```python
from build123d import *

# Parameters (mm, degrees)
SKETCH1_R            = 8.6
BOSS_EXTRUDE11_DEPTH = 5
SKETCH20_R           = 8.6
BOSS_EXTRUDE12_DEPTH = 5
SKETCH21_R           = 8.55
BOSS_EXTRUDE13_DEPTH = 1
SKETCH22_R           = 8.55
BOSS_EXTRUDE14_DEPTH = 7.5
SKETCH24_R           = 2.15
CUT_EXTRUDE8_DEPTH   = 7
BOSS_EXTRUDE15_START = 11.25
SKETCH30_R           = 8.55
BOSS_EXTRUDE15_DEPTH = 11.25
SKETCH31_R           = 1.6
CUT_EXTRUDE12_DEPTH  = 29.75
SKETCH32_R           = 1.5
CUT_EXTRUDE13_DEPTH  = 22.75
CIRPATTERN7_COUNT    = 2
CIRPATTERN8_COUNT    = 2
SKETCH33_R           = 2.1
CUT_EXTRUDE14_DEPTH  = 5.8
CUT_EXTRUDE15_DEPTH  = 3


with BuildPart() as part:
    # Sketch1 → Boss-Extrude11 (new body)
    with BuildSketch(Plane(origin=(0, 0, 0), x_dir=(1, 0, 0), z_dir=(0, 1, 0))):
        with Locations(Location((0, 0, 0), (0, 0, 270))):
            Circle(SKETCH1_R)
    extrude(amount=BOSS_EXTRUDE11_DEPTH)

    # Sketch20 → Boss-Extrude12 (add)
    with BuildSketch(Plane(origin=(0, 5, 0), x_dir=(1, 0, 0), z_dir=(0, 1, 0))):
        with Locations(Location((1, 0, 0), (0, 0, 93.333029494))):
            Circle(SKETCH20_R)
    extrude(amount=BOSS_EXTRUDE12_DEPTH)

    # Sketch21 → Boss-Extrude13 (add)
    with BuildSketch(Plane(origin=(0, 10, 0), x_dir=(1, 0, 0), z_dir=(0, 1, 0))):
        with Locations(Location((0.5, 0, 0), (0, 0, 94.074449123))):
            Circle(SKETCH21_R)
    extrude(amount=BOSS_EXTRUDE13_DEPTH)

    # Sketch22 → Boss-Extrude14 (add)
    with BuildSketch(Plane(origin=(0, 11, 0), x_dir=(1, 0, 0), z_dir=(0, 1, 0))):
        with Locations(Location((0.5, 0, 0), (0, 0, 94.074449123))):
            Circle(SKETCH22_R)
    extrude(amount=BOSS_EXTRUDE14_DEPTH)

    # Sketch24 → Cut-Extrude8 (cut)
    with BuildSketch(Plane(origin=(0, 18.5, 0), x_dir=(1, 0, 0), z_dir=(0, 1, 0))):
        with Locations(Location((0.7, 5, 0), (0, 0, 270))):
            Circle(SKETCH24_R)
    cut_extrude8 = extrude(amount=-CUT_EXTRUDE8_DEPTH, mode=Mode.SUBTRACT)

    # Sketch30 → Boss-Extrude15 (add)
    with BuildSketch(Plane.XZ.offset(BOSS_EXTRUDE15_START)):
        with Locations(Location((0.5, 0, 0), (0, 0, 265.925550877))):
            Circle(SKETCH30_R)
    extrude(amount=-BOSS_EXTRUDE15_DEPTH)

    # Sketch31 → Cut-Extrude12 (cut)
    with BuildSketch(Plane(origin=(0, 18.5, 0), x_dir=(1, 0, 0), z_dir=(0, 1, 0))):
        with Locations(Location((6.7, 0, 0), (0, 0, 270))):
            Circle(SKETCH31_R)
    cut_extrude12 = extrude(amount=-CUT_EXTRUDE12_DEPTH, mode=Mode.SUBTRACT)

    # Sketch32 → Cut-Extrude13 (cut)
    with BuildSketch(Plane(origin=(0, 11.5, 0), x_dir=(1, 0, 0), z_dir=(0, 1, 0))):
        with Locations(Location((0.7, 5, 0), (0, 0, 270))):
            Circle(SKETCH32_R)
    cut_extrude13 = extrude(amount=-CUT_EXTRUDE13_DEPTH, mode=Mode.SUBTRACT)

    # CirPattern7: Cut-Extrude12 ×2 about axis
    cirpattern7_axis = Axis((0.5, 0, 0), (0, 1, 0))
    for i in range(1, CIRPATTERN7_COUNT):
        add(cut_extrude12.rotate(cirpattern7_axis, i * 360 / CIRPATTERN7_COUNT), mode=Mode.SUBTRACT)

    # CirPattern8: Cut-Extrude8, Cut-Extrude13 ×2 about axis
    cirpattern8_axis = Axis((0.5, 0, 0), (0, 1, 0))
    add([cut_extrude8.rotate(cirpattern8_axis, i * 360 / CIRPATTERN8_COUNT) for i in range(1, CIRPATTERN8_COUNT)], mode=Mode.SUBTRACT)
    add([cut_extrude13.rotate(cirpattern8_axis, i * 360 / CIRPATTERN8_COUNT) for i in range(1, CIRPATTERN8_COUNT)], mode=Mode.SUBTRACT)

    # Sketch33 → Cut-Extrude14 (cut)
    with BuildSketch(Plane.XZ.offset(11.25)):
        with Locations(Location((0.7, 0, 0), (0, 0, 270))):
            Circle(SKETCH33_R)
    extrude(amount=-CUT_EXTRUDE14_DEPTH, mode=Mode.SUBTRACT)

    # Sketch34 → Cut-Extrude15 (cut)
    with BuildSketch(Plane(origin=(0, 18.5, 0), x_dir=(1, 0, 0), z_dir=(0, 1, 0))):
        with BuildLine():
            Line((-5.7, 3), (-9.054437868, 3))
            Line((-9.054437868, 3), (-9.054437868, -2.973683702))
            Line((-9.054437868, -2.973683702), (-5.30350884, -2.973683702))
            ThreePointArc((-5.30350884, -2.973683702), (-2.706586304, 0.198681773), (-5.7, 3))
        make_face()
        with BuildLine():
            Line((6.7, 3), (10.113600604, 3))
            Line((10.113600604, 3), (10.113600604, -3))
            Line((10.113600604, -3), (6.7, -3))
            ThreePointArc((6.7, -3), (3.7, 0), (6.7, 3))
        make_face()
    extrude(amount=-CUT_EXTRUDE15_DEPTH, mode=Mode.SUBTRACT)


solid = part.part
```
The listing builds one solid part. Answer for the finished solid, in the listing's coordinates (mm). A direction names the side the tool comes from. Round coordinates to 2 decimals unless told otherwise and drop trailing zeros. Loops run counter-clockwise (first coordinate to the right, second up) from the corner with the lowest first, then second, coordinate; pieces in that order, holes last. Notation, with made-up numbers: (49.25, 64.25) -> (53.25, 64.25) arc R23 cw to (53.25, 74.25) -> close; hole circle Ø5 at (33, -12.75). An arc over 180 degrees is marked (long way). Use one line per item in the form item = value.
1. Find the intervals of material crossed by probe 1 along X at (y, z) = (-9.3, 0); probe 2 along X at (y, z) = (8.75, 0); probe 3 along Z at (x, y) = (0.25, 13.25), in increasing order. Write a range as [from, to].
Answer key:
probe_1 = [-8.05, -7.3], [-4.1, -1.4], [2.8, 5.1], [8.3, 9.05]
probe_2 = [-7.6, -7.3], [-4.1, 5.1], [8.3, 9.6]
probe_3 = [-8.55, -7.1], [-2.9, 2.85], [7.15, 8.55]
2. For a pull along X with two mould halves and no side action, classify faces 1 (the cylindrical face through (1.71, 0.28, -6.11)), 2 (the flat face through (-7, 17, -3)), 3 (the cylindrical face through (3.21, 14.19, -8.11)) as released by +X, released by -X, zero draft, split by the parting line, or undercut.
Answer key:
face_1 = undercut
face_2 = zero draft
face_3 = split by the parting line
3. The part is cut by section D-D on y = -7.5. Determine the outline of the cut face in (x, z), and give its area (3 significant figures).
Answer key:
outline = circle Ø17.1 at (0.5, 0); hole circle Ø3.2 at (-5.7, 0); hole circle Ø4.2 at (0.7, 0); hole circle Ø3 at (0.3, 5); hole circle Ø3 at (0.7, -5); hole circle Ø3.2 at (6.7, 0)
area = 186 mm²
4. The part is cut by section C-C on z = -5. Determine the outline of the cut face in (x, y).
Answer key:
outline = (-7, 0) -> (-6.44, 0) -> (-6.44, -11.25) -> (-0.8, -11.25) -> (-0.8, 11.5) -> (-1.45, 11.5) -> (-1.45, 18.5) -> (-6.44, 18.5) -> (-6.44, 10) -> (-6, 10) -> (-6, 5) -> (-7, 5) -> close; (2.2, -11.25) -> (7.44, -11.25) -> (7.44, 0) -> (7, 0) -> (7, 5) -> (8, 5) -> (8, 10) -> (7.44, 10) -> (7.44, 18.5) -> (2.85, 18.5) -> (2.85, 11.5) -> (2.2, 11.5) -> close
5. The part is cut by section B-B on y = -2.5. Determine the outline of the cut face in (x, z), and give its area (3 significant figures).
Answer key:
outline = circle Ø17.1 at (0.5, 0); hole circle Ø3.2 at (-5.7, 0); hole circle Ø3 at (0.3, 5); hole circle Ø3 at (0.7, -5); hole circle Ø3.2 at (6.7, 0)
area = 199 mm²
6. Flat-ended cylindrical pins translate along their axes: pin 1 Ø4 at (y, z) = (9.5, 5) entering from +X; pin 2 Ø4 at (x, y) = (-6, -8) entering from -Z; pin 3 Ø0.7 at (x, y) = (-6.5, 17.5) entering from -Z. Find the tip coordinate at first contact, or state that the pin passes through.
Answer key:
pin_1 = 9.06
pin_2 = -7.27
pin_3 = -5.37
7. The part is cut by section A-A on z = 0. Give the number of separate pieces and of enclosed holes in the cut face, and give its area (3 significant figures).
Answer key:
separate_pieces = 3
enclosed_holes = 0
area = 282 mm²
8. A tool of negligible diameter and unlimited length cuts with its end or side. For faces 4 (the cylindrical face through (3.7, 17, 0.1)), 5 (the flat face through (1, -5.45, 0)), 6 (the cylindrical face through (-5.233, 2.465, -6.825)), 7 (the flat face through (-7.9, 10, 0)), 8 (the cylindrical face through (0.21, 15.05, 7.15)), from which of +Z, -Z, +X, -X, +Y, -Y can it reach the whole face along a straight path? Write none if from no direction.
Answer key:
face_4 = +X, +Y
face_5 = -Y
face_6 = none
face_7 = -X
face_8 = +Y
